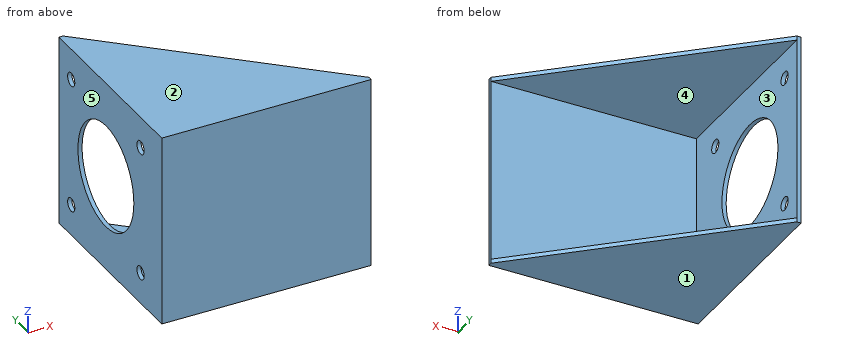
from build123d import *

# Parameters (mm, degrees)
EXTRUDE_1_DEPTH     = 46
EXTRUDE_2_DEPTH     = 1
EXTRUDE_3_DEPTH     = 1
SKETCH_5_R          = 1.6
SKETCH_5_R_2        = 12.5
CUT_EXTRUDE_1_DEPTH = 1


with BuildPart() as part:
    # 草图2 → 凸台-拉伸1 (new body)
    with BuildSketch(Plane.XY):
        Polygon((0, 46), (0, 0), (50, 0), (50, 1), (1, 1), (1, 46), align=None)
    extrude(amount=EXTRUDE_1_DEPTH)

    # 草图3 → 凸台-拉伸2 (add)
    with BuildSketch(Plane.XY.offset(46)):
        Polygon((1, 46), (50, 1), (1, 1), align=None)
    extrude(amount=-EXTRUDE_2_DEPTH)

    # 草图4 → 凸台-拉伸3 (add)
    with BuildSketch(Plane(origin=(0, 0, 0), x_dir=(-1, 0, 0), z_dir=(0, 0, -1))):
        Polygon((-1, 46), (-50, 1), (-1, 1), align=None)
    extrude(amount=-EXTRUDE_3_DEPTH)

    # 草图5 → 切除-拉伸1 (cut)
    with BuildSketch(Plane.ZY):
        with Locations(Location((7.5, 40.5, 0), (0, 0, 270))):
            Circle(SKETCH_5_R)
        with Locations(Location((38.5, 40.5, 0), (0, 0, 90))):
            Circle(SKETCH_5_R)
        with Locations(Location((7.5, 9.5, 0), (0, 0, 270))):
            Circle(SKETCH_5_R)
        with Locations(Location((38.5, 9.5, 0), (0, 0, 90))):
            Circle(SKETCH_5_R)
        with Locations(Location((23, 25, 0), (0, 0, 270))):
            Circle(SKETCH_5_R_2)
    extrude(amount=-CUT_EXTRUDE_1_DEPTH, mode=Mode.SUBTRACT)


solid = part.part
Geometry: final body of the model. Coordinates: model frame, mm. Face numbers are marked on the shaded views. A direction names the side the tool comes from. Coordinates: 2 decimals unless noted, no trailing zeros. Order: outer loops, then holes, each group sorted by start corner. A loop starts at its lowest first (then second) coordinate and runs counter-clockwise, first axis right, second up.
(1) Section query D-D (y = 40.5). Return the cut outline in (x, z), plus the area to 3 significant figures.
(2) First-contact query: pin 1 (3 mm diameter, centred on y = 40.5, z = 7.5, fed in from -X); pin 2 (2 mm diameter, centred on x = 35, z = 33.5, fed in from +Y); pin 3 (22 mm diameter, centred on y = 14, z = 24, fed in from +X). Flat tips, straight axial feed; report the tip coordinate or a pass-through.
(3) Draft query along Z for the marked faces 1, 2 and 3. Return one class per face: pulls with the +Z half, pulls with the -Z half, needs draft (parallel to the pull), parting line crosses it, or undercut.
(4) Section query C-C (z = 38.5). Return the cut outline in (x, y), plus the area to 3 significant figures.
(5) Material intervals for probe 1 along Z at (x, y) = (0.65, 40.5); probe 2 along Y at (x, z) = (0.35, 38.5); probe 3 along Z at (x, y) = (38.5, 2.5), sorted ascending.
(6) Section query B-B (y = 25). Return the cut outline in (x, z), plus the area to 3 significant figures.
(7) Access query for the marked faces 4 and 5. Directions: +Z, -Z, +X, -X, +Y, -Y. A direction counts if a zero-diameter tool reaches every point of the face in a straight line with its end or side. Return the directions, or none.
(8) Section query A-A (z = 23). Return the cut outline in (x, y), plus the area to 3 significant figures.
Solution:
1. outline: (0, 0) - (6.99, 0) - (6.99, 1) - (1, 1) - (1, 5.9) - (0, 5.9) - close; (0, 9.1) - (1, 9.1) - (1, 36.9) - (0, 36.9) - close; (0, 40.1) - (1, 40.1) - (1, 45) - (6.99, 45) - (6.99, 46) - (0, 46) - close
1. area: 51.6 mm2
2. pin 1: passes through
2. pin 2: stops at y = 1
2. pin 3: stops at x = 1
3. face 1: pulls with the -Z half
3. face 2: pulls with the +Z half
3. face 3: undercut
4. outline: (0, 0) - (50, 0) - (50, 1) - (1, 1) - (1, 7.9) - (0, 7.9) - close; (0, 11.1) - (1, 11.1) - (1, 38.9) - (0, 38.9) - close; (0, 42.1) - (1, 42.1) - (1, 46) - (0, 46) - close
4. area: 88.6 mm2
5. probe 1: z = 0 to 5.9, 9.1 to 36.9, 40.1 to 46
5. probe 2: y = 0 to 7.9, 11.1 to 38.9, 42.1 to 46
5. probe 3: z = 0 to 1, 45 to 46
6. outline: (0, 0) - (23.87, 0) - (23.87, 1) - (1, 1) - (1, 10.5) - (0, 10.5) - close; (0, 35.5) - (1, 35.5) - (1, 45) - (23.87, 45) - (23.87, 46) - (0, 46) - close
6. area: 66.7 mm2
7. face 4: +X, +Y
7. face 5: +Z, -Z, -X, +Y, -Y
8. outline: (0, 0) - (50, 0) - (50, 1) - (1, 1) - (1, 12.5) - (0, 12.5) - close; (0, 37.5) - (1, 37.5) - (1, 46) - (0, 46) - close
8. area: 70.0 mm2
